Source: CAD feature listing. Evaluate the final solid. Frame: model axes, mm. Face numbers are marked on the shaded views. A direction names the side the tool comes from. Give positions to 0.01 mm unless a question says otherwise; leave off trailing zeros. Write each loop counter-clockwise with the first axis right and the second up, starting at its lowest first coordinate (ties: lowest second). Pieces come first, ordered by that corner, then holes. Notation, with made-up numbers: (45.5, -9) - (51.5, -9) arc R33 ccw to (51.5, 30) - close; hole circle Ø3 at (6, -39.75). An arc over 180 degrees is marked (long way). Answer as a JSON object with one key per item and string values. Group by question number.
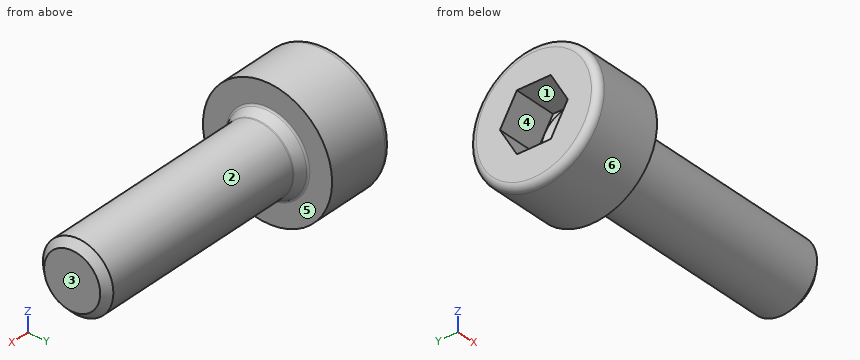
Autodesk Inventor part; units mm, degrees
ref_plane "IP1_XY" through (0, 0, 0) normal (1, 0, 0) x (0, 0, -1)
ref_plane "IP1_YZ" through (0, 0, 0) normal (0, 0, -1) x (0, 1, 0)
ref_plane "IP1_ZX" through (0, 0, 0) normal (0, 1, 0) x (1, 0, 0)
sketch "Skizze_2" plane through (0, 0, 0) normal (0, 0, 1) x (1, 0, 0)
  line L0 (10, 0) -> (-0.4283, 0)
  line L1 (-0.4283, 0) -> (-1.15, 1.25)
  line L2 (-1.15, 1.25) -> (-3, 1.25)
  line L3 (-3, 1.25) -> (-3, 2.45)
  arc A0 (-2.7, 2.75) -> (-3, 2.45) centre (-2.7, 2.45) ccw
  line L4 (-2.7, 2.75) -> (0, 2.75)
  line L5 (0, 2.75) -> (0, 1.8)
  arc A1 (0, 1.8) -> (0.0562, 1.7101) centre (0.1, 1.8) ccw
  line L6 (0.0562, 1.7101) -> (0.4662, 1.5101)
  arc A2 (0.4662, 1.5101) -> (0.51, 1.5) centre (0.51, 1.6) ccw
  line L7 (0.51, 1.5) -> (9.6935, 1.5)
  line L8 (9.6935, 1.5) -> (10, 1.1935)
  line L9 (10, 1.1935) -> (10, 0)
  line L10 (10, 0) -> (-0.4283, 0)
revolve "Revolution1" add sketch "Skizze_2" angle 360 about axis through (10, 0, 0) along (1, 0, 0)
thread "Thread1"
sketch "Skizze_1" plane through (-1.15, 0, 0) normal (1, 0, 0) x (0, 0, -1)
  line L0 (-1.25, -0.7217) -> (0, -1.4434)
  line L1 (0, -1.4434) -> (1.25, -0.7217)
  line L2 (1.25, -0.7217) -> (1.25, 0.7217)
  line L3 (1.25, 0.7217) -> (0, 1.4434)
  line L4 (0, 1.4434) -> (-1.25, 0.7217)
  line L5 (-1.25, 0.7217) -> (-1.25, -0.7217)
extrude "Extrusion1" cut sketch "Skizze_1" against normal blind 2.6
ref_plane "IP1_XY" through (0, 0, 0) normal (1, 0, 0) x (0, 0, -1)
ref_plane "IP1_YZ" through (0, 0, 0) normal (0, 0, -1) x (0, 1, 0)
ref_plane "IP1_ZX" through (0, 0, 0) normal (0, 1, 0) x (1, 0, 0)
ref_plane "IP2_XY" through (-3, 0, 0) normal (1, 0, 0) x (0, 0, -1)
ref_plane "IP2_YZ" through (-3, 0, 0) normal (0, 0, -1) x (0, 1, 0)
ref_plane "IP2_ZX" through (-3, 0, 0) normal (0, 1, 0) x (1, 0, 0)
ref_plane "IP3_XY" through (10, 0, 0) normal (1, 0, 0) x (0, 0, -1)
ref_plane "IP3_YZ" through (10, 0, 0) normal (0, 0, -1) x (0, 1, 0)
ref_plane "IP3_ZX" through (10, 0, 0) normal (0, 1, 0) x (1, 0, 0)
ref_plane "IP4_XY" through (0, 0, 0) normal (1, 0, 0) x (0, 0, -1)
ref_plane "IP4_YZ" through (0, 0, 0) normal (0, 0, -1) x (0, 1, 0)
ref_plane "IP4_ZX" through (0, 0, 0) normal (0, 1, 0) x (1, 0, 0)
properties part number "Slotted head cap screw ISO 4762 - M3x10" material "鋼、炭素鋼"
Q1. First-contact query: pin 1 Ø1 at (x, y) = (6.5, 1.5) entering from +Z; pin 2 Ø0.7 at (y, z) = (-1, 0) entering from -X; pin 3 Ø1 at (y, z) = (1, 1.5) entering from +X. Flat tips, straight axial feed; report the tip coordinate or a pass-through.
Q2. Section A-A on x = 4.25. Return the cut outline in (y, z).
Q3. Ray query, probe 1 along X at (y, z) = (2.25, -0.45); probe 2 along Z at (x, y) = (4.5, 0.05); probe 3 along Y at (x, z) = (7, -1.35). Return the intervals inside material, ascending. Write a range as [from, to].
Q4. Reachability of the marked faces 5 and 6 from +Z, -Z, +X, -X, +Y, -Y: full face, straight path, thin tool, end or side. Return the list, or none.
Q5. Draft query along Z for the marked faces 1, 2, 3 and 4. Return one class per face: released by +Z, released by -Z, zero draft, split by the parting line, or undercut.
Taken from the geometry:
{
 "1": {"pin 1": "stops at z = 1.12", "pin 2": "stops at x = -1.15", "pin 3": "stops at x = 9.89"},
 "2": {"outline": "circle Ø3 at (0, 0)"},
 "3": {"probe 1": "x = [-3, 0]", "probe 2": "z = [-1.5, 1.5]", "probe 3": "y = [-0.65, 0.65]"},
 "4": {"face 5": "+X", "face 6": "+X, -X"},
 "5": {"face 1": "undercut", "face 2": "split by the parting line", "face 3": "zero draft", "face 4": "undercut"}
}
